Can you work these out from the model? Positions are in its coordinate system, mm. Face numbers are marked on the shaded views. Coordinates: 2 decimals unless noted, no trailing zeros. Order: outer loops, then holes, each group sorted by start corner. A loop starts at its lowest first (then second) coordinate and runs counter-clockwise, first axis right, second up. Notation, with made-up numbers: (59, -28.5) - (114, -28.5) arc R28 ccw to (114, 0.5) - close; hole circle Ø4 at (45, -34.75). An arc over 180 degrees is marked (long way). Return JSON: item names as keys, results as strings. Group by question number.
1) Imagine slicing it at D-D (z = 42.75). Write out the boundary of the cut face in (x, y), and give its area (3 significant figures).
2) If I drill on line 1 along Z through (x, y) = (-23.5, -2.75); line 2 along Z through (x, y) = (-25, -2.4); line 3 along X through (y, z) = (-0.95, 45.5), over which ranges is the centre line in solid material (lowest first)?
3) Imagine slicing it at C-C (z = 45.5). Write out the boundary of the cut face in (x, y), and give its area (3 significant figures).
4) If we mould it in two halves opening along Z, with no side actions, what happens to the marked faces 1, 2, 3 and 4? For each: pulls with the +Z half, pulls with the -Z half, needs draft (parallel to the pull), parting line crosses it, or undercut.
5) For pin 1 Ø2 at (x, y) = (-17.5, -0.5) entering from +Z; pin 2 Ø3 at (x, y) = (-18, -1.5) entering from +Z; pin 3 Ø3 at (x, y) = (-16.5, -3) entering from +Z, each with a flat end and sliding along its axis, tell me the tip position at first contact or that it passes through.
6) Imagine slicing it at A-A (x = -21.5). Write out the boundary of the cut face in (y, z).
```python
from build123d import *

# Parameters (mm, degrees)
F0_R     = 3.175
F1_DEPTH = 5


with BuildPart() as f1:
    # F0 (on Front) → F1 (new body)
    with BuildSketch(Plane.XZ):
        with BuildLine():
            ThreePointArc((-13.347524, 37.588448), (-12.461887, 36.712299), (-11.659195, 35.759579))
            Line((-11.659195, 35.759579), (-10.344394, 40.666482))
            Line((-10.344394, 40.666482), (-26.876474, 56.333769))
            Line((-26.876474, 56.333769), (-29.725796, 58.255821))
            Line((-29.725796, 58.255821), (-29.725796, 44.399414))
            Line((-29.725796, 44.399414), (-26.876474, 43.988798))
            Line((-26.876474, 43.988798), (-17.436201, 41.282147))
            Line((-17.436201, 41.282147), (-13.347524, 37.588448))
        make_face()
        with Locations((-24.010796, 47.518508)):
            Circle(F0_R, mode=Mode.SUBTRACT)
    extrude(amount=F1_DEPTH)


solid = f1.part
```
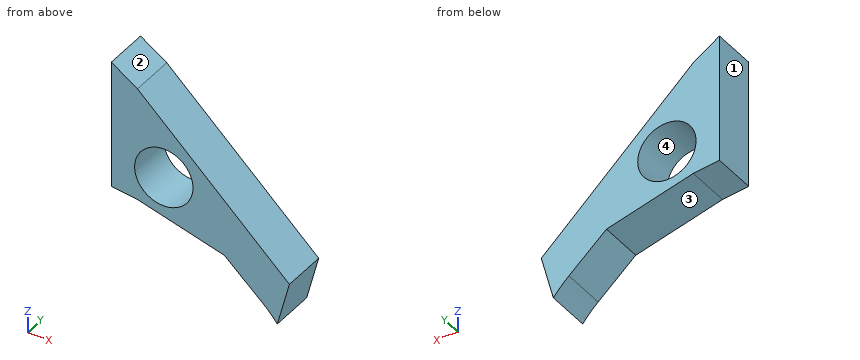
Calculated:
{
 "1": {"outline": "(-22.56, -5) - (-12.54, -5) - (-12.54, 0) - (-22.56, 0) - close", "area": "50.1 mm2"},
 "2": {"line 1": "43.02 to 44.38, 50.65 to 53.13", "line 2": "43.45 to 44.5, 50.54 to 54.56", "line 3": "-29.73 to -26.46, -21.56 to -15.44"},
 "3": {"outline": "(-29.73, -5) - (-26.46, -5) - (-26.46, 0) - (-29.73, 0) - close; (-21.56, -5) - (-15.44, -5) - (-15.44, 0) - (-21.56, 0) - close", "area": "46.9 mm2"},
 "4": {"face 1": "needs draft", "face 2": "pulls with the +Z half", "face 3": "pulls with the -Z half", "face 4": "undercut"},
 "5": {"pin 1": "z = 48.4", "pin 2": "z = 49.34", "pin 3": "z = 47.92"},
 "6": {"outline": "(-5, 42.45) - (0, 42.45) - (0, 45.58) - (-5, 45.58) - close; (-5, 49.46) - (0, 49.46) - (0, 51.24) - (-5, 51.24) - close"}
}
